from build123d import *

# Parameters (mm, degrees)
SKETCH_3_W          = 12
SKETCH_3_H          = 12
CUT_EXTRUDE_1_DEPTH = 3
FILLET_1_R          = 1.5


with BuildPart() as part:
    # 草图1 → 放样1 section 0
    with BuildSketch(Plane.XY):
        with BuildLine():
            Line((-9, -9), (9, -9))
            Line((9, -9), (9, 9))
            Line((9, 9), (-9, 9))
            Line((-9, 9), (-9, -9))
        make_face()
    # 草图2 → 放样1 section 1
    with BuildSketch(Plane.XY.offset(8)):
        with BuildLine():
            Line((-7, -7), (7, -7))
            Line((7, -7), (7, 7))
            Line((7, 7), (-7, 7))
            Line((-7, 7), (-7, -7))
        make_face()
    loft()

    # 草图3 → 切除-拉伸1 (cut)
    with BuildSketch(Plane.XY):
        Rectangle(SKETCH_3_W, SKETCH_3_H)
    extrude(amount=CUT_EXTRUDE_1_DEPTH, mode=Mode.SUBTRACT)

    # 圆角1
    fillet_1_edges = [part.edges().sort_by_distance(p)[0] for p in [
        (0, 7, 8),
        (7, 0, 8),
        (0, -7, 8),
        (-7, 0, 8),
    ]]
    fillet(fillet_1_edges, radius=FILLET_1_R)


solid = part.part
The listing builds one solid part. Answer for the finished solid, in the listing's coordinates (mm). A direction names the side the tool comes from. Give positions to 0.01 mm unless a question says otherwise; leave off trailing zeros. Put each result on its own line as item: value.
Item 1: Straight lines are drawn through the part: line 1 (Y direction, x = -1.75, z = 1); line 2 (Y direction, x = -0.25, z = 2); line 3 (Z direction, x = 0.5, y = 4.75). For each, find the intervals that lie inside material, in ascending order.
Established:
line 1: y = -8.75 to -6, 6 to 8.75
line 2: y = -8.5 to -6, 6 to 8.5
line 3: z = 3 to 8
Item 2: For a pull along Y with two mould halves and no side action, classify faces 1 (the face through (0, 0, 8)), 2 (the face through (0, -6, 1)) as released by +Y, released by -Y, zero draft, split by the parting line, or undercut.
Established:
face 1: zero draft
face 2: undercut
Item 3: Given P1, Ø0.9, axis at y = 0.5, z = 1, coming from the +X side; P2, Ø1.5, axis at x = -0.5, z = 1.5, coming from the -Y side; P3, Ø3.5, axis at x = 2, z = 2, coming from the +Y side, each flat-ended and moving along its own axis, determine where each tip first touches the part or whether it passes through.
Established:
P1: stops at x = 8.86
P2: stops at y = -8.81
P3: stops at y = 8.94
Item 4: For faces 3 (the face through (-6, 0, 1)), 4 (the face through (7, -1, 0)), determine the directions among +Z, -Z, +X, -X, +Y, -Y from which every point of the face is accessible in a straight line to the end or side of a thin tool.
Established:
face 3: -Z
face 4: -Z, +X, -X, +Y, -Y
